from build123d import *

# Parameters (mm, degrees)
F0_W     = 108
F0_H     = 60
F1_DEPTH = 7
F3_DEPTH = 5
F4_R     = 1.75
F5_DEPTH = 7.001
F7_DEPTH = 3
F8_R     = 1.75
F9_DEPTH = 3
F10_R    = 1


with BuildPart() as f1:
    # F0 (on Top) → F1 (new body)
    with BuildSketch(Plane.XY):
        Rectangle(F0_W, F0_H)
    extrude(amount=F1_DEPTH)

    # F2 (on face) → F3 (join)
    with BuildSketch(Plane.XY.offset(7)):
        Polygon((54, 30), (-54, 30), (-54, -30), (54, -30), (54, -27), (51, -27), (-51, -27), (-51, 27), (51, 27), (54, 27), align=None)
    extrude(amount=F3_DEPTH)

    # F4 (on face) → F5 (cut, through all)
    with BuildSketch(Plane.XY.offset(7)):
        with Locations((-45.75, 24.25)):
            Circle(F4_R)
        with Locations((39.75, 24.25)):
            Circle(F4_R)
    extrude(amount=-F5_DEPTH, mode=Mode.SUBTRACT)

    # F6 (on face) → F7 (cut)
    with BuildSketch(Plane(origin=(0, 0, 0), x_dir=(1, 0, 0), z_dir=(0, 0, -1))):
        Polygon((35.625, -21.8684301396), (35.625, -26.6315698604), (39.75, -29.0131397208), (43.875, -26.6315698604), (43.875, -21.8684301396), (39.75, -19.4868602792), align=None)
        Polygon((-49.875, -21.8684301396), (-49.875, -26.6315698604), (-45.75, -29.0131397208), (-41.625, -26.6315698604), (-41.625, -21.8684301396), (-45.75, -19.4868602792), align=None)
    extrude(amount=-F7_DEPTH, mode=Mode.SUBTRACT)

    # F8 (on Top) → F9 (join)
    with BuildSketch(Plane.XY):
        with BuildLine():
            Line((10, -30), (-10, -30))
            ThreePointArc((-10, -30), (0, -39.928586731), (10, -30))
        make_face()
        with Locations((0, -34.1783299042)):
            Circle(F8_R, mode=Mode.SUBTRACT)
        with BuildLine():
            Line((-10, 30), (10, 30))
            ThreePointArc((10, 30), (0, 40.0551036455), (-10, 30))
        make_face()
        with Locations((0, 34.25)):
            Circle(F8_R, mode=Mode.SUBTRACT)
    extrude(amount=F9_DEPTH)

    # F10
    f10_edges = [f1.edges().sort_by_distance(p)[0] for p in [
        (54, 0, 0),
        (32, -30, 0),
        (0, -39.928587, 0),
        (-54, 0, 0),
        (-32, 30, 0),
        (0, 40.055104, 0),
        (32, 30, 0),
    ]]
    fillet(f10_edges, radius=F10_R)


solid = f1.part
Source: CAD feature listing. Evaluate the final solid. Frame: model axes, mm. A direction names the side the tool comes from. Give positions to 0.01 mm unless a question says otherwise; leave off trailing zeros. Loops run counter-clockwise (first coordinate to the right, second up) from the corner with the lowest first, then second, coordinate; pieces in that order, holes last. Notation, with made-up numbers: (81, 39) -> (122, 39) arc R13 ccw to (122, 52) -> close; hole circle Ø7 at (55, -17.75). An arc over 180 degrees is marked (long way). Use a Markdown table: item, result. Add a question column.
1) Section query C-C, the plane y = 9. Return the cut outline in (x, z).
2) Reachability of faces 4 (the face through (-41.625, 24, 1)), 5 (the face through (1.669, 34.776, 1.479)), 6 (the face through (-51, 0, 9)), 7 (the face through (-0.219, -39.926, 1.986)), 8 (the face through (2, -34, 3)) from +Z, -Z, +X, -X, +Y, -Y: full face, straight path, thin tool, end or side. Return the list, or none.
3) Pull-direction query (X, two-part tool) for faces 1 (the face through (37.659, 27.806, 1.479)), 2 (the face through (-1, -30, 6)), 3 (the face through (0.221, 40.053, 1.986)); classes: +X half, -X half, draft (parallel to the pull), parting line (faces both ways), or undercut.
4) Section query A-A, the plane z = 4.5. Return the cut outline in (x, y), then the cut area to 3 significant figures.
5) Section query B-B, the plane x = 0. Return the cut outline in (y, z), then the cut area to 3 significant figures.
6) First-contact query: pin 1 (4 mm diameter, centred on x = 0, y = 34.25, fed in from +Z); pin 2 (5 mm diameter, centred on y = -30.5, z = 3.5, fed in from -X); pin 3 (6 mm diameter, centred on x = -14.5, z = 3.5, fed in from -Y); pin 4 (5.5 mm diameter, centred on x = 27, z = 10, fed in from +Y). Flat tips, straight axial feed; report the tip coordinate or a pass-through.
7) Line query: line 1 along Y through (x, z) = (0, 1.95); line 2 along X through (y, z) = (24, 6.5); line 3 along Y through (x, z) = (-18, 8.5). Output: solid intervals per line, ascending. Write a range as [from, to].
8) Section query D-D, the plane x = -33.5. Return the cut outline in (y, z), then the cut area to 3 significant figures.
Numbers:
| question | item | result |
|---|---|---|
| 1 | outline | (-54, 1) arc R1 ccw to (-53, 0) -> (53, 0) arc R1 ccw to (54, 1) -> (54, 7) -> (-51, 7) -> (-51, 12) -> (-54, 12) -> close |
| 2 | face 4 | -Z |
| 2 | face 5 | +Z, -Z |
| 2 | face 6 | +Z, +X |
| 2 | face 7 | +Z, -Z, -Y |
| 2 | face 8 | +Z, +X, -X, -Y |
| 3 | face 1 | undercut |
| 3 | face 2 | draft |
| 3 | face 3 | parting line |
| 4 | outline | (-54, -30) -> (54, -30) -> (54, 30) -> (-54, 30) -> close; hole circle Ø3.5 at (-45.75, 24.25); hole circle Ø3.5 at (39.75, 24.25) |
| 4 | area | 6,460 mm2 |
| 5 | outline | (-39.93, 1) arc R1 ccw to (-38.93, 0) -> (-35.93, 0) -> (-35.93, 3) -> (-39.93, 3) -> close; (-32.43, 0) -> (32.5, 0) -> (32.5, 3) -> (30, 3) -> (30, 12) -> (27, 12) -> (27, 7) -> (-27, 7) -> (-27, 12) -> (-30, 12) -> (-30, 3) -> (-32.43, 3) -> close; (36, 0) -> (39.06, 0) arc R1 ccw to (40.06, 1) -> (40.06, 3) -> (36, 3) -> close |
| 5 | area | 489 mm2 |
| 6 | pin 1 | stops at z = 3 |
| 6 | pin 2 | stops at x = -54 |
| 6 | pin 3 | stops at y = -30 |
| 6 | pin 4 | stops at y = 30 |
| 7 | line 1 | y = [-39.93, -35.93], [-32.43, 32.5], [36, 40.06] |
| 7 | line 2 | x = [-54, -47.48], [-44.02, 38.02], [41.48, 54] |
| 7 | line 3 | y = [-30, -27], [27, 30] |
| 8 | outline | (-30, 0) -> (29, 0) arc R1 ccw to (30, 1) -> (30, 12) -> (27, 12) -> (27, 7) -> (-27, 7) -> (-27, 12) -> (-30, 12) -> close |
| 8 | area | 450 mm2 |
